The model under review builds one solid part; all positions refer to its coordinate system, in mm. Round coordinates to 2 decimals unless told otherwise and drop trailing zeros. Answer as a JSON object with one key per item and string values. Group by question number.
1) To check wall thickness, follow line 1 (Z direction, x = -12, y = 45); line 2 (Z direction, x = 31, y = 26.5); line 3 (Y direction, x = -22.5, z = 12.25). State the ranges of each line that lie inside material, in increasing order.
2) Insertion check: pin 1 Ø8 at (y, z) = (13.5, 20) entering from -X; pin 2 Ø1 at (y, z) = (-8, 5) entering from -X; pin 3 Ø5 at (x, z) = (-41, 6.5) entering from -Y (3 decimals); pin 4 Ø4 at (x, z) = (-37, 8) entering from +Y. Each pin has a flat end and moves straight along its axis. Give the tip position at first contact, or say it passes through.
3) The part is to be moulded in two halves that separate along X. For faces 1 (the flat face through (-66.019, 18, 13)), 2 (the flat face through (2, 50.8, 1)), 3 (the cylindrical face through (-39.571, -1.892, 13.803)), say which applies: +X half, -X half, draft (parallel to the pull), parting line (faces both ways), or undercut.
```python
from build123d import *

# Parameters (mm, degrees)
F2_DEPTH      = 25.4
F2_DEPTH_BACK = 50.8
F3_DEPTH      = 25.4


with BuildPart() as f2:
    # F1 (on Front) → F2 (new body, two sides)
    with BuildSketch(Plane.XZ) as f2_sk:
        with BuildLine():
            add(Edge.make_bspline(
                [(-66.493101418, 0), (-31.6023416817, 4.5892358758), (0, 4.5892358758), (67.7957311273, 0)],
                knots=[0, 0, 0, 0, 134.2888325453, 134.2888325453, 134.2888325453, 134.2888325453], degree=3))
            Line((-66.493101418, 0), (67.7957311273, 0))
        make_face()
    extrude(amount=F2_DEPTH)
    extrude(f2_sk.sketch, amount=-F2_DEPTH_BACK)

    # F0 (on Top) → F3 (join)
    with BuildSketch(Plane.XY):
        with BuildLine():
            add(Edge.make_bspline(
                [(-66.0190582275, 15.8042479306), (-50.882216543, 15.443845652), (-44.3860767732, 10.0356803936), (-41.1722754867, -0.5532574777)],
                knots=[0, 0, 0, 0, 29.7477830393, 29.7477830393, 29.7477830393, 29.7477830393], degree=3))
            ThreePointArc((-41.1722754867, -0.5532574777), (-39.5395729632, -1.8954823631), (-37.6727509093, -0.9043917556))
            add(Edge.make_bspline(
                [(-37.6727509093, -0.9043917556), (-35.9554500646, 2.279277761), (-11.7834584129, 13.3395817627), (10.1645017819, 9.6475739081), (63.7337581556, -1.8624929201)],
                knots=[0, 0, 0, 0, 0.3222291325, 1, 1, 1, 1], degree=3))
            ThreePointArc((63.7337581556, -1.8624929201), (65.9847645302, -0.4510784554), (64.6355761504, 1.8377664946))
            add(Edge.make_bspline(
                [(-66.0190582275, 19.8427634791), (-18.4567762815, 21.7484285157), (11.260919046, 16.4069097143), (64.6355761504, 1.8377664946)],
                knots=[0, 0, 0, 0, 131.8893983641, 131.8893983641, 131.8893983641, 131.8893983641], degree=3))
            Line((-66.0190582275, 19.8427634791), (-66.0190582275, 15.8042479306))
        make_face()
    extrude(amount=F3_DEPTH)


solid = f2.part
```
Results list:
{
 "1": {"line 1": "0 to 3.44", "line 2": "0 to 2.21", "line 3": "7.34 to 19.23"},
 "2": {"pin 1": "x = -66.02", "pin 2": "through", "pin 3": "y = -1.905", "pin 4": "y = 20.09"},
 "3": {"face 1": "-X half", "face 2": "draft", "face 3": "undercut"}
}
